Build history of the part. All positions in model axes, mm. A direction names the side the tool comes from. Round coordinates to 2 decimals unless told otherwise and drop trailing zeros. Order: outer loops, then holes, each group sorted by start corner. A loop starts at its lowest first (then second) coordinate and runs counter-clockwise, first axis right, second up. Notation, with made-up numbers: (84.25, 20) -> (112.25, 20) arc R15 ccw to (112.25, 39) -> close; hole circle Ø1 at (6, 58). An arc over 180 degrees is marked (long way). Use a Markdown table: item, result. Add a question column.
Item 1: Slice it at A-A, the plane y = 6. Give the cut face in (x, z), plus the area to 3 significant figures.
Item 2: Slice it at C-C, the plane x = 10.5. Give the cut face in (y, z), plus the area to 3 significant figures.
Item 3: Pin check, flat tips, straight feed: pin 1 (4 mm diameter, centred on x = 34.5, y = 12, fed in from +Z); pin 2 (5 mm diameter, centred on y = 36, z = 44.5, fed in from -X); pin 3 (12 mm diameter, centred on x = 13.5, z = 39.5, fed in from -Y). Stop position of each tip, or through.
Item 4: 3-axis set-ups, long thin cutter, end or side, ignore diameter. For faces 5 (the face through (19, 50, 25)), 6 (the face through (45, 35, 38)), 7 (the face through (35, 20, 5)): which of +Z, -Z, +X, -X, +Y, -Y reach the whole face in a straight line?
Item 5: Probe L1, parallel to Z at x = 33, y = 32; L2, parallel to X at y = 21, z = 21.5; L3, parallel to X at y = 24.5, z = 20. List the from-to ranges inside material, lowest first.
Item 6: Slice it at D-D, the plane y = 11. Give the cut face in (x, z).
Item 7: Two-plate mould, pull along X, no slides. Class faces 1 (the face through (28, 30, 15)), 2 (the face through (36, 14, 25)), 3 (the face through (50, 30, 19)), 4 (the face through (27.3, 39, 25)): released by +X, released by -X, zero draft, split by the parting line, or undercut.
Item 8: Slice it at B-B, the plane z = 23. Give the cut face in (x, y).
from build123d import *

# Parameters (mm, degrees)
F0_W      = 50
F0_H      = 50
F1_DEPTH  = 50
F2_W      = 20
F2_H      = 10
F3_DEPTH  = 30
F8_DEPTH  = 35
F10_DEPTH = 25
F12_REACH = 115.9479483752


with BuildPart() as f1:
    # F0 (on Top) → F1 (new body)
    with BuildSketch(Plane.XY):
        with Locations((25, 25)):
            Rectangle(F0_W, F0_H)
    extrude(amount=F1_DEPTH)

    # F2 (on face) → F3 (cut)
    with BuildSketch(Plane.YZ.offset(50)):
        with Locations((30, 5)):
            Rectangle(F2_W, F2_H)
    extrude(amount=-F3_DEPTH, mode=Mode.SUBTRACT)

    # F7 (on face) → F8 (cut)
    with BuildSketch(Plane.XY.offset(50)):
        Polygon((15, 0), (50, 50), (35, 50), (0, 0), align=None)
    extrude(amount=-F8_DEPTH, mode=Mode.SUBTRACT)

    # F9 (on face) → F10 (cut)
    with BuildSketch(Plane.XY.offset(50)):
        Polygon((15, 0), (50, 0), (50, 35), (39.5, 35), align=None)
    extrude(amount=-F10_DEPTH, mode=Mode.SUBTRACT)

    f12_end = Plane(origin=(37.75, 32.5, 27.5), x_dir=(-0.5734623444, -0.8192319205, 0), z_dir=(-0.8192319205, 0.5734623444, 0))
    # F11 (on face) → F12 (cut, up to a plane its end follows)
    with BuildSketch(Plane(origin=(0, 0, 0), x_dir=(0, -1, 0), z_dir=(-1, 0, 0))):
        Polygon((0, 50), (-50, 50), (0, 7), align=None)
    f12_long = extrude(amount=-F12_REACH, mode=Mode.PRIVATE)
    add(split(f12_long, bisect_by=f12_end, keep=Keep.TOP, mode=Mode.PRIVATE), mode=Mode.SUBTRACT)


solid = f1.part
Check sheet entries:
| question | item | result |
|---|---|---|
| 1 | outline | (0, 0) -> (50, 0) -> (50, 25) -> (19.2, 25) -> (19.2, 12.16) -> (0, 12.16) -> close |
| 1 | area | 1,000 mm2 |
| 2 | outline | (0, 0) -> (50, 0) -> (50, 50) -> (15, 19.9) -> (15, 15) -> (9.3, 15) -> (0, 7) -> close |
| 2 | area | 1,410 mm2 |
| 3 | pin 1 | z = 25 |
| 3 | pin 2 | x = 39.5 |
| 3 | pin 3 | y = 30.81 |
| 4 | face 5 | +Z, -Z, +X, -X, +Y |
| 4 | face 6 | +Z, +X, -Y |
| 4 | face 7 | -Z, +X |
| 5 | L1 | 10 to 15 |
| 5 | L2 | 0 to 14.7, 29.7 to 50 |
| 5 | L3 | 0 to 17.15, 32.15 to 50 |
| 6 | outline | (0, 0) -> (50, 0) -> (50, 25) -> (22.7, 25) -> (22.7, 15) -> (7.7, 15) -> (7.7, 16.46) -> (0, 16.46) -> close |
| 7 | face 1 | undercut |
| 7 | face 2 | zero draft |
| 7 | face 3 | released by +X |
| 7 | face 4 | undercut |
| 8 | outline | (0, 18.6) -> (13.02, 18.6) -> (35, 50) -> (0, 50) -> close; (15, 0) -> (50, 0) -> (50, 50) -> close |
